The listing builds one solid part. Answer for the finished solid, in the listing's coordinates (mm). A direction names the side the tool comes from. Coordinates: 2 decimals unless noted, no trailing zeros. Order: outer loops, then holes, each group sorted by start corner. A loop starts at its lowest first (then second) coordinate and runs counter-clockwise, first axis right, second up. Notation, with made-up numbers: (28.25, -37) -> (65.25, -37) arc R20 ccw to (65.25, -11) -> close; hole circle Ø1 at (-13, 31.5). An arc over 180 degrees is marked (long way). Answer in a Markdown table with one row per item.
Autodesk Inventor part; units mm, degrees
ref_plane "YZ Plane" through (0, 0, 0) normal (1, 0, 0) x (0, 1, 0)
ref_plane "XZ Plane" through (0, 0, 0) normal (0, 1, 0) x (-1, 0, 0)
ref_plane "XY Plane" through (0, 0, 0) normal (0, 0, 1) x (1, 0, 0)
sketch "Sketch1" plane through (0, 0, 0) normal (0, 0, 1) x (1, 0, 0)
  line L0 (0, 0) -> (209.2, 0)
  line L1 (209.2, 0) -> (209.2, 119.3)
  line L2 (209.2, 119.3) -> (0, 119.3)
  line L3 (0, 119.3) -> (0, 0)
  dimension "d0" = 209.2
  dimension "d1" = 119.3
extrude "Extrusion1" add sketch "Sketch1" along normal blind 10
fillet "Fillet1" radius 12 4 edges at (209.2, 119.3, 5) (209.2, 0, 5) (0, 119.3, 5) (0, 0, 5)
sketch "Sketch3" plane through (0, 0, 10) normal (0, 0, 1) x (1, 0, 0)
  circle A0 centre (18, 101.602) radius 3.5
  line L0 (0, 107.3) -> (0, 12)
  line L1 (197.2, 119.3) -> (12, 119.3)
  line L2 (197.2, 119.3) -> (12, 119.3) construction
  line L3 (104.6, 119.3) -> (104.6, 0) construction
  line L4 (12, 0) -> (197.2, 0) construction
  circle A1 centre (191.2, 101.602) radius 3.5
  line L5 (0, 59.65) -> (209.2, 59.65) construction
  line L6 (209.2, 12) -> (209.2, 107.3) construction
  circle A2 centre (18, 17.698) radius 3.5
  circle A3 centre (191.2, 17.698) radius 3.5
  point P0 (0, 0)
  dimension "d16" = 7
  dimension "d17" = 18
  dimension "d18" = 17.698
extrude "Extrusion3" cut sketch "Sketch3" against normal through all
sketch "Sketch4" plane through (0, 0, 10) normal (0, 0, 1) x (1, 0, 0)
  circle A0 centre (18, 101.602) radius 3.5 construction
  line L0 (18, 101.602) -> (18, 119.3) construction
  line L1 (12, 119.3) -> (24, 119.3)
  arc A1 (12, 119.3) -> (0, 107.3) centre (12, 107.3) ccw
  line L2 (0, 107.3) -> (0, 95.3)
  line L3 (197.2, 119.3) -> (12, 119.3) construction
  line L4 (104.6, 119.3) -> (104.6, 0) construction
  line L5 (12, 0) -> (197.2, 0) construction
  line L6 (0, 107.3) -> (0, 12) construction
  line L7 (0, 59.65) -> (209.2, 59.65) construction
  line L8 (209.2, 12) -> (209.2, 107.3) construction
  line L9 (191.2, 101.602) -> (191.2, 119.3) construction
  line L10 (197.2, 119.3) -> (185.2, 119.3)
  arc A2 (209.2, 107.3) -> (197.2, 119.3) centre (197.2, 107.3) ccw
  line L11 (209.2, 107.3) -> (209.2, 95.3)
  line L12 (12, 0) -> (24, 0)
  arc A3 (0, 12) -> (12, 0) centre (12, 12) ccw
  line L13 (0, 12) -> (0, 24)
  line L14 (197.2, 0) -> (12, 0) construction
  line L15 (197.2, 0) -> (185.2, 0)
  line L16 (209.2, 12) -> (209.2, 24)
  arc A4 (197.2, 0) -> (209.2, 12) centre (197.2, 12) ccw
  line L17 (24, 0) -> (185.2, 0)
  line L18 (0, 95.3) -> (0, 24)
  line L19 (209.2, 93.9155) -> (209.2, 24)
  line L20 (209.2, 12) -> (209.2, 107.3)
  line L21 (197.2, 119.3) -> (12, 119.3)
  line L22 (24, 119.3) -> (197.2, 119.3)
  point P0 (0, 0)
  point P1 (104.6, 107.3)
  point P2 (12, 59.65)
  point P3 (18, 17.698)
  point P4 (191.2, 17.698)
  dimension "d21" = 12
  dimension "d22" = 12
extrude "Extrusion4" cut sketch "Sketch4" against normal blind 10 keep common part
sketch "Sketch5" plane through (0, 0, 10) normal (0, 0, 1) x (1, 0, 0)
  line L0 (43.891, 114.602) -> (165.309, 114.602)
  line L1 (43.891, 4.698) -> (165.309, 4.698)
  line L2 (12, 0) -> (197.2, 0)
  line L3 (104.6, 107.3) -> (104.6, 0) construction
  line L4 (43.891, 114.602) -> (5, 75.7075)
  line L5 (5, 43.5925) -> (5, 75.7075)
  line L6 (5, 43.5925) -> (43.891, 4.698)
  line L7 (165.309, 114.602) -> (204.2, 75.7075)
  line L8 (204.2, 43.5925) -> (204.2, 75.7075)
  line L9 (204.2, 43.5925) -> (165.309, 4.698)
  line L10 (0, 107.3) -> (0, 12)
  line L11 (0, 59.65) -> (209.2, 59.65) construction
  line L12 (209.2, 12) -> (209.2, 107.3) construction
  line L13 (197.2, 119.3) -> (12, 119.3) construction
  point P0 (0, 0)
  point P1 (104.6, 114.602)
  point P2 (5, 59.65)
  dimension "d25" = 4.698
  dimension "d27" = 121.418
  dimension "d37" = 5
  dimension "d38" = 32.115
  dimension "d39" = 4.698
extrude "Extrusion5" cut sketch "Sketch5" against normal through all
sketch "Sketch8" plane through (0, 0, 10) normal (0, 0, 1) x (1, 0, 0)
  line L0 (197.2, 119.3) -> (12, 119.3)
  line L1 (12, 119.3) -> (197.2, 119.3)
  line L2 (209.2, 12) -> (209.2, 107.3)
  line L3 (209.2, 107.3) -> (209.2, 12)
  line L4 (12, 0) -> (197.2, 0)
  line L5 (197.2, 0) -> (12, 0)
  line L6 (0, 107.3) -> (0, 12)
  line L7 (0, 107.3) -> (0, 12)
  arc A0 (12, 119.3) -> (0, 107.3) centre (12, 107.3) ccw
  arc A1 (209.2, 107.3) -> (197.2, 119.3) centre (197.2, 107.3) ccw
  arc A2 (197.2, 0) -> (209.2, 12) centre (197.2, 12) ccw
  arc A3 (0, 12) -> (12, 0) centre (12, 12) ccw
  line L8 (5, 75.7075) -> (5, 12)
  line L9 (5, 75.7075) -> (5, 107.3)
  line L10 (165.309, 4.698) -> (43.891, 4.698)
  line L11 (43.891, 4.698) -> (12, 4.698)
  line L12 (165.309, 4.698) -> (197.2, 4.698)
  line L13 (204.2, 43.5925) -> (204.2, 75.7075)
  line L14 (204.2, 75.7075) -> (204.2, 12)
  line L15 (204.2, 75.7075) -> (204.2, 107.3)
  line L16 (43.891, 114.602) -> (197.2, 114.602)
  line L17 (43.891, 114.602) -> (165.309, 114.602)
  line L18 (43.891, 114.602) -> (12, 114.602)
  arc A4 (5, 12) -> (12, 4.698) centre (12.3085, 12) ccw
  arc A5 (197.2, 4.698) -> (204.2, 12) centre (196.8915, 12) ccw
  arc A6 (204.2, 107.3) -> (197.2, 114.602) centre (197.2, 107.5958) ccw
  arc A7 (12, 114.602) -> (5, 107.3) centre (12, 107.5958) ccw
  point P0 (0, 0)
extrude "Extrusion7" add sketch "Sketch8" along normal blind 60
properties part number "THAD Back"
(1) A cutting plane is placed at A-A, the plane x = 50.5. Determine the outline of the cut face in (y, z), then the cut area to 3 significant figures.
Check values:
| item | result |
|---|---|
| outline | (0, 0) -> (4.7, 0) -> (4.7, 70) -> (0, 70) -> close; (114.6, 0) -> (119.3, 0) -> (119.3, 70) -> (114.6, 70) -> close |
| area | 658 mm² |
(2) Which of the six approach directions +Z, -Z, +X, -X, +Y, -Y give full straight-line access (tool end or side, diameter ignored) to faces 4 (the cylindrical face through (6.9, 112.4, 39.6)), 5 (the flat face through (184.48, 95.43, 5.07)), 6 (the cylindrical face through (3.61, 3.42, 34.51))?
Check values:
| item | result |
|---|---|
| face 4 | +Z |
| face 5 | +Z, -Z |
| face 6 | +Z, -Z, -X, -Y |
(3) Find the intervals of material crossed by line 1 along Y through (x, z) = (114.5, 55); line 2 along X through (y, z) = (77.5, 66.5); line 3 along Y through (x, z) = (191.2, 3), in increasing order. Write a range as from..to.
Check values:
| item | result |
|---|---|
| line 1 | 0..4.7, 114.6..119.3 |
| line 2 | 0..5, 204.2..209.2 |
| line 3 | 0..14.2, 21.2..30.59, 88.71..98.1, 105.1..119.3 |
(4) A cutting plane is placed at D-D, the plane x = 18. Determine the outline of the cut face in (y, z).
Check values:
| item | result |
|---|---|
| outline | (0, 0) -> (14.2, 0) -> (14.2, 10) -> (4.7, 10) -> (4.7, 70) -> (0, 70) -> close; (21.2, 0) -> (30.59, 0) -> (30.59, 10) -> (21.2, 10) -> close; (88.71, 0) -> (98.1, 0) -> (98.1, 10) -> (88.71, 10) -> close; (105.1, 0) -> (119.3, 0) -> (119.3, 70) -> (114.6, 70) -> (114.6, 10) -> (105.1, 10) -> close |
(5) A cutting plane is placed at C-C, the plane y = 46.5. Determine the outline of the cut face in (x, z), then the cut area to 3 significant figures.
Check values:
| item | result |
|---|---|
| outline | (0, 0) -> (5, 0) -> (5, 70) -> (0, 70) -> close; (204.2, 0) -> (209.2, 0) -> (209.2, 70) -> (204.2, 70) -> close |
| area | 700 mm² |
(6) For a pull along X with two mould halves and no side action, classify faces 1 (the flat face through (0, 60, 35)), 2 (the flat face through (209.2, 59, 35)), 3 (the flat face through (103, 114.602, 35)) as released by +X, released by -X, zero draft, split by the parting line, or undercut.
Check values:
| item | result |
|---|---|
| face 1 | released by -X |
| face 2 | released by +X |
| face 3 | undercut |
(7) A cutting plane is placed at B-B, the plane z = 28. Determine the outline of the cut face in (x, y), then the cut area to 3 significant figures.
Check values:
| item | result |
|---|---|
| outline | (0, 12) arc R12 ccw to (12, 0) -> (197.2, 0) arc R12 ccw to (209.2, 12) -> (209.2, 107.3) arc R12 ccw to (197.2, 119.3) -> (12, 119.3) arc R12 ccw to (0, 107.3) -> close; hole (5, 12) arc R7.31 ccw to (12, 4.7) -> (197.2, 4.7) arc R7.31 ccw to (204.2, 12) -> (204.2, 107.3) arc R7.01 ccw to (197.2, 114.6) -> (12, 114.6) arc R7.01 ccw to (5, 107.3) -> close |
| area | 2,980 mm² |
(8) Flat-ended cylindrical pins translate along their axes: pin 1 (4 mm diameter, centred on x = 191.2, y = 101.602, fed in from -Z); pin 2 (11 mm diameter, centred on x = 191.2, y = 17.698, fed in from +Z). Find the tip coordinate at first contact, or state that the pin passes through.
Check values:
| item | result |
|---|---|
| pin 1 | through |
| pin 2 | z = 10 |
